Autodesk Fusion 360 part; units mm, degrees
sketch "Sketch1" plane through (0, 0, 0) normal (0, 0, 1) x (1, 0, 0)
  line L0 (21, 0) -> (21, 3.8)
  line L1 (21, 3.8) -> (7, 3.8)
  line L2 (7, 3.8) -> (7, 0)
  line L3 (17, 0) -> (17, 1.4)
  line L4 (17, 1.4) -> (11, 1.4)
  line L5 (11, 1.4) -> (11, 0)
  line L6 (0, 57.2) -> (68.8, 57.2) construction
  line L7 (34.4, 114.4) -> (34.4, 0) construction
  line L8 (47.8, 0) -> (47.8, 3.8)
  line L9 (47.8, 3.8) -> (61.8, 3.8)
  line L10 (61.8, 3.8) -> (61.8, 0)
  line L11 (51.8, 1.4) -> (57.8, 1.4)
  line L12 (57.8, 1.4) -> (57.8, 0)
  line L13 (51.8, 0) -> (51.8, 1.4)
  line L14 (7, 110.6) -> (7, 114.4)
  line L15 (21, 110.6) -> (7, 110.6)
  line L16 (21, 114.4) -> (21, 110.6)
  line L17 (17, 113) -> (11, 113)
  line L18 (11, 113) -> (11, 114.4)
  line L19 (17, 114.4) -> (17, 113)
  line L20 (47.8, 114.4) -> (47.8, 110.6)
  line L21 (47.8, 110.6) -> (61.8, 110.6)
  line L22 (51.8, 113) -> (57.8, 113)
  line L23 (51.8, 114.4) -> (51.8, 113)
  line L24 (57.8, 113) -> (57.8, 114.4)
  line L25 (61.8, 110.6) -> (61.8, 114.4)
  line L26 (68.8, 54.2) -> (67.4, 54.2)
  line L27 (67.4, 54.2) -> (67.4, 60.2)
  line L28 (67.4, 60.2) -> (68.8, 60.2)
  line L29 (68.8, 50.2) -> (65, 50.2)
  line L30 (65, 50.2) -> (65, 64.2)
  line L31 (65, 64.2) -> (68.8, 64.2)
  line L32 (3.8, 64.2) -> (0, 64.2)
  line L33 (3.8, 50.2) -> (3.8, 64.2)
  line L34 (0, 50.2) -> (3.8, 50.2)
  line L35 (0, 54.2) -> (1.4, 54.2)
  line L36 (1.4, 54.2) -> (1.4, 60.2)
  line L37 (1.4, 60.2) -> (0, 60.2)
  line L38 (7, 0) -> (11, 0)
  line L39 (17, 0) -> (21, 0)
  line L40 (0, 0) -> (11, 0)
  line L41 (17, 0) -> (51.8, 0)
  line L42 (57.8, 0) -> (68.8, 0)
  line L43 (68.8, 0) -> (68.8, 54.2)
  line L44 (68.8, 60.2) -> (68.8, 114.4)
  line L45 (68.8, 64.2) -> (68.8, 60.2)
  line L46 (68.8, 54.2) -> (68.8, 50.2)
  line L47 (0, 114.4) -> (0, 60.2)
  line L48 (0, 54.2) -> (0, 0)
  line L49 (11, 114.4) -> (0, 114.4)
  line L50 (68.8, 114.4) -> (57.8, 114.4)
  line L51 (51.8, 114.4) -> (17, 114.4)
  line L52 (18.6, 1.6) -> (50.2, 1.6)
  line L53 (50.2, 1.6) -> (50.2, 3)
  line L54 (50.2, 3) -> (59.4, 3)
  line L55 (59.4, 3) -> (59.4, 1.6)
  line L56 (59.4, 1.6) -> (67.2, 1.6)
  line L57 (67.2, 1.6) -> (67.2, 52.6)
  line L58 (67.2, 52.6) -> (65.8, 52.6)
  line L59 (65.8, 52.6) -> (65.8, 61.8)
  line L60 (65.8, 61.8) -> (67.2, 61.8)
  line L61 (67.2, 61.8) -> (67.2, 112.8)
  line L62 (67.2, 112.8) -> (59.4, 112.8)
  line L63 (18.6, 1.6) -> (18.6, 3)
  line L64 (18.6, 3) -> (9.4, 3)
  line L65 (9.4, 3) -> (9.4, 1.6)
  line L66 (8.5, 1.6) -> (9.4, 1.6)
  line L67 (1.6, 52.6) -> (1.6, 1.6)
  line L68 (1.6, 1.6) -> (9.4, 1.6)
  line L69 (1.6, 52.6) -> (3, 52.6)
  line L70 (3, 52.6) -> (3, 61.8)
  line L71 (3, 61.8) -> (1.6, 61.8)
  line L72 (1.6, 112.8) -> (1.6, 61.8)
  line L73 (67.2, 112.8) -> (59.4, 112.8)
  line L74 (59.4, 111.4) -> (59.4, 112.8)
  line L75 (50.2, 111.4) -> (59.4, 111.4)
  line L76 (50.2, 112.8) -> (50.2, 111.4)
  line L77 (50.2, 112.8) -> (18.6, 112.8)
  line L78 (18.6, 112.8) -> (18.6, 111.4)
  line L79 (18.6, 111.4) -> (9.4, 111.4)
  line L80 (9.4, 111.4) -> (9.4, 112.8)
  line L81 (9.4, 112.8) -> (1.6, 112.8)
  line L82 (22.6, 114.4) -> (22.6, 109)
  line L83 (22.6, 109) -> (5.4, 109)
  line L84 (5.4, 109) -> (5.4, 114.4)
  line L85 (46.2, 114.4) -> (46.2, 109)
  line L86 (46.2, 109) -> (63.4, 109)
  line L87 (63.4, 109) -> (63.4, 114.4)
  line L88 (68.8, 48.6) -> (63.4, 48.6)
  line L89 (63.4, 48.6) -> (63.4, 65.8)
  line L90 (63.4, 65.8) -> (68.8, 65.8)
  line L91 (46.2, 0) -> (46.2, 5.4)
  line L92 (46.2, 5.4) -> (63.4, 5.4)
  line L93 (63.4, 5.4) -> (63.4, 0)
  line L94 (22.6, 0) -> (22.6, 5.4)
  line L95 (22.6, 5.4) -> (5.4, 5.4)
  line L96 (5.4, 5.4) -> (5.4, 0)
  line L97 (0, 48.6) -> (5.4, 48.6)
  line L98 (5.4, 48.6) -> (5.4, 65.8)
  line L99 (5.4, 65.8) -> (0, 65.8)
  line L100 (1.6, 29.4948) -> (3.6, 29.4948)
  line L101 (3.6, 29.4948) -> (3.6, 26.4948)
  line L102 (3.6, 26.4948) -> (1.6, 26.4948)
  line L103 (1.6, 26.4948) -> (1.6, 29.4948)
  line L104 (67.2, 29.4948) -> (65.2, 29.4948)
  line L105 (65.2, 29.4948) -> (65.2, 26.4948)
  line L106 (65.2, 26.4948) -> (67.2, 26.4948)
  line L107 (67.2, 84.9052) -> (65.2, 84.9052)
  line L108 (65.2, 84.9052) -> (65.2, 87.9052)
  line L109 (65.2, 87.9052) -> (67.2, 87.9052)
  line L110 (3.6, 84.9052) -> (3.6, 87.9052)
  line L111 (1.6, 84.9052) -> (3.6, 84.9052)
  line L112 (3.6, 87.9052) -> (1.6, 87.9052)
  line L113 (28.4, 112.8) -> (31.4, 112.8)
  line L114 (31.4, 112.8) -> (31.4, 110.8)
  line L115 (31.4, 110.8) -> (28.4, 110.8)
  line L116 (28.4, 110.8) -> (28.4, 112.8)
  line L117 (28.4, 3.6) -> (28.4, 1.6)
  line L118 (31.4, 3.6) -> (28.4, 3.6)
  line L119 (31.4, 1.6) -> (31.4, 3.6)
  line L120 (37.4, 110.8) -> (40.4, 110.8)
  line L121 (40.4, 110.8) -> (40.4, 112.8)
  line L122 (37.4, 112.8) -> (37.4, 110.8)
  line L123 (37.4, 1.6) -> (37.4, 3.6)
  line L124 (37.4, 3.6) -> (40.4, 3.6)
  line L125 (40.4, 3.6) -> (40.4, 1.6)
  point P0 (14, 0)
  point P1 (14, 0)
  point P2 (7, 0)
  point P3 (14, 0)
  point P4 (68.8, 50.2)
  dimension "d10" = 68.8
  dimension "d11" = 114.4
  dimension "d12" = 14
  dimension "d13" = 7
  dimension "d14" = 3
  dimension "d15" = 14
  dimension "d16" = 3.8
  dimension "d17" = 6
  dimension "d18" = 1.4
  dimension "d19" = 3
  dimension "d20" = 7
  dimension "d21" = 1.4
  dimension "d22" = 6
  dimension "d23" = 3.8
  dimension "d24" = 14
  dimension "d30" = -1.6
  dimension "d31" = 1.6
  dimension "d32" = -1.6
  dimension "d33" = -1.6
  dimension "d34" = 1.6
  dimension "d35" = 1.6
  dimension "d36" = 2
  dimension "d37" = 3
  dimension "d38" = 3
  dimension "d39" = 2
  dimension "d40" = 6
extrude "Extrude1" add sketch "Sketch1" along normal blind 4.2 contours L0 L41 L52 L94 | L41 L52 L91 L94 | L8 L41 L52 L91 | L52 L117 L118 L119 | L2 L40 L68 L96 | L52 L123 L124 L125 | L40 L48 L67 L68 L96 L97 L103 | L10 L42 L56 L93 | L42 L43 L56 L57 L88 L93 | L34 L48 L67 L97 | L29 L43 L57 L88 | L47 L49 L72 L81 L84 L99 | L32 L47 L72 L99 | L31 L44 L61 L90 | L44 L50 L61 L62 L73 L87 L90 | L14 L49 L81 L84 | L25 L50 L62 L73 L87 | L51 L77 L82 L85 L113 | L16 L51 L77 L82 | L77 L113 L114 L115 L116 | L20 L51 L77 L85 | L77 L120 L121 L122 makes body 1 at (29.9333, 0, 2.8) makes body 2 at (68.8, 16.7333, 2.8) makes body 3 at (0, 33.4667, 2.8) makes body 4 at (38.8667, 114.4, 1.4) makes body 5 at (68.8, 80.9333, 1.4) makes body 6 at (0, 97.6667, 1.4)
extrude "Extrude2" add sketch "Sketch1" along normal blind 1.8 contours L0 L2 L3 L4 L5 L38 L39 L40 L41 L52 L63 L64 L65 L66 L68 | L0 L1 L2 L52 L63 L64 L65 L66 L68 | L8 L10 L11 L12 L13 L41 L42 L52 L53 L54 L55 L56 | L8 L9 L10 L52 L53 L54 L55 L56 | L32 L34 L35 L36 L37 L47 L48 L67 L69 L70 L71 L72 | L32 L33 L34 L67 L69 L70 L71 L72 | L26 L27 L28 L29 L31 L43 L44 L45 L46 L57 L58 L59 L60 L61 | L29 L30 L31 L57 L58 L59 L60 L61 | L14 L16 L17 L18 L19 L49 L51 L77 L78 L79 L80 L81 | L14 L15 L16 L77 L78 L79 L80 L81 | L20 L22 L23 L24 L25 L50 L51 L62 L73 L74 L75 L76 L77 | L20 L21 L25 L62 L73 L74 L75 L76 L77 bodies 1 5 2 4 3 6
fillet "Fillet1" radius 2 4 edges at (7, 112.8, 0.9) (21, 112.8, 0.9) (47.8, 112.8, 0.9) (61.8, 112.8, 0.9) on bodies 1
fillet "Fillet1" radius 2 8 edges at (61.8, 1.6, 0.9) (21, 1.6, 0.9) (67.2, 64.2, 0.9) (47.8, 1.6, 0.9) (7, 1.6, 0.9) (67.2, 50.2, 0.9) (1.6, 50.2, 0.9) (1.6, 64.2, 0.9) on bodies 1
ref_plane "WorkPlane1" through (0, 57.2, 0) normal (0, 1, 0) x (0, 0, 1)
equation "width = 68.8 mm"
equation "height = 114.4 mm"
equation "depth = 4.2 mm"
equation "inner_depth = 1.6 mm"
equation "insets_width = 14 mm"
equation "insets_height = 3.8 mm"
equation "insets_niche_depth = 1.4 mm"
equation "insets_niche_width = 6 mm"
equation "insets_topbot_center_from_edge = 14 mm"
equation "d10 = width"
equation "d11 = height"
equation "d12 = insets_topbot_center_from_edge"
equation "d13 = insets_width / 2"
equation "d14 = insets_niche_width / 2"
equation "d15 = insets_width"
equation "d16 = insets_height"
equation "d17 = insets_niche_width"
equation "d18 = insets_niche_depth"
equation "d19 = insets_niche_width / 2"
equation "d20 = insets_width / 2"
equation "d21 = insets_niche_depth"
equation "d22 = insets_niche_width"
equation "d23 = insets_height"
equation "d24 = insets_width"
equation "d41 = depth"
equation "d49 = height / 2"
Here's how the part is built. I have some questions about the finished solid (model axes, mm). A direction names the side the tool comes from. Round coordinates to 2 decimals unless told otherwise and drop trailing zeros. Order: outer loops, then holes, each group sorted by start corner. A loop starts at its lowest first (then second) coordinate and runs counter-clockwise, first axis right, second up. Notation, with made-up numbers: M 71,73.25 L 95,73.25 A8 cw 95,86.25 Z; hole C -25.5,81 d2. An arc over 180 degrees is marked long. One line per question, with ' | ' between items.
1) For pin 1 Ø1.4 at (x, z) = (12, 0.5) entering from -Y; pin 2 Ø4 at (x, y) = (10, 112.5) entering from +Z, each with a flat end and sliding along its axis, tell me the tip position at first contact or that it passes through.
Working result:
pin 1: y = 1.4 | pin 2: z = 1.8
2) I want a section at B-B, the plane x = 38.5. Write out the boundary of the cut face in (y, z), then the cut area to 3 significant figures.
Working result:
outline: M 0,0 L 3.6,0 L 3.6,4.2 L 0,4.2 Z; M 110.8,0 L 114.4,0 L 114.4,4.2 L 110.8,4.2 Z | area: 30.2 mm²
3) I need wall thicknesses on line 1 along X through (y, z) = (75.5, 2.2); line 2 along Y through (x, z) = (23, 1.2); line 3 along Y through (x, z) = (14, 0.9). Which ranges of each line are inside material? Lowest first, please.
Working result:
line 1: 0 to 1.6, 67.2 to 68.8 | line 2: 0 to 1.6, 112.8 to 114.4 | line 3: 1.4 to 3.8, 110.6 to 113
4) For faces 1 (the face through (34, 1.6, 2)), 2 (the face through (1, 93, 4.2)), 3 (the face through (4, 112.8, 2)), which set-ups out of +Z, -Z, +X, -X, +Y, -Y let a thin tool reach every point of the face, with its end or its side?
Working result:
face 1: +Z, -Z | face 2: +Z, +X, -X, +Y, -Y | face 3: +Z
5) I want a section at A-A, the plane y = 92.5. Write out the boundary of the cut face in (x, z), then the cut area to 3 significant figures.
Working result:
outline: M 0,0 L 1.6,0 L 1.6,4.2 L 0,4.2 Z; M 67.2,0 L 68.8,0 L 68.8,4.2 L 67.2,4.2 Z | area: 13.4 mm²
6) I want a section at C-C, the plane z = 2.9. State how many separate pieces and enclosed holes the cut face has, then the cut area to 3 significant figures.
Working result:
separate pieces: 6 | enclosed holes: 0 | area: 466 mm²
7) If we mould it in two halves opening along X, with no side actions, what happens to faces 4 (the face through (1, 62, 0)), 5 (the face through (0, 27, 2)), 6 (the face through (65, 1.6, 2))? For each: +X half, -X half, draft (parallel to the pull), parting line (faces both ways), or undercut.
Working result:
face 4: draft | face 5: -X half | face 6: undercut
